Here's the drawing with two shaded views (mm, measured from the low corner). I have some questions. A direction names the side the tool comes from. Give positions to 0.01 mm unless a question says otherwise; leave off trailing zeros. Loops run counter-clockwise (first coordinate to the right, second up) from the corner with the lowest first, then second, coordinate; pieces in that order, holes last. Notation, with made-up numbers: (39.25, 31) - (92.25, 31) arc R21 cw to (92.25, 59) - close; hole circle Ø6 at (68.5, 85.5). An arc over 180 degrees is marked (long way). Use one line per item in the form item = value.
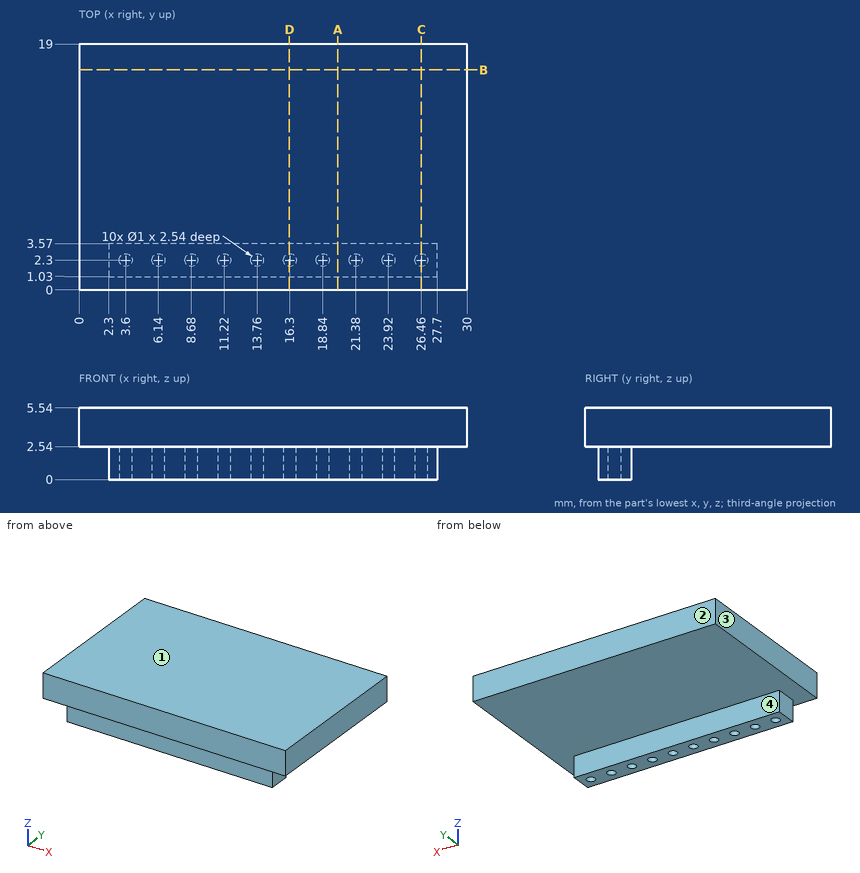
(1) For the marked faces 3 and 4, which set-ups out of +Z, -Z, +X, -X, +Y, -Y let a thin tool reach every point of the face, with its end or its side?
Geometry says:
face_3 = +Z, -Z, -X, +Y, -Y
face_4 = -Z, +X, -X, +Y
(2) If I drill on probe 1 along Y at (x, z) = (13.75, 1.15); probe 2 along Z at (x, y) = (14.75, 7); probe 3 along Y at (x, z) = (23.25, 1.85), over which ranges is the centre line in solid material (lowest first)?
Geometry says:
probe_1 = 1.03 to 1.8, 2.8 to 3.57
probe_2 = 2.54 to 5.54
probe_3 = 1.03 to 3.57
(3) For P1, Ø3, axis at x = 20.5, z = 1, coming from the -Y side; P2, Ø2, axis at y = 1.5, z = 1, coming from the -X side; P3, Ø0.8, axis at x = 10.5, z = 0.5, coming from the +Y side, each with a flat end and sliding along its axis, tell me the tip position at first contact or that it passes through.
Geometry says:
P1 = 1.03
P2 = 2.3
P3 = 3.57
(4) If we section it at C-C (x = 26.46): List the corners of the cut face in (y, z) for me.
Geometry says:
outline = (0, 2.54) - (1.03, 2.54) - (1.03, 0) - (1.8, 0) - (1.8, 2.54) - (2.8, 2.54) - (2.8, 0) - (3.57, 0) - (3.57, 2.54) - (19, 2.54) - (19, 5.54) - (0, 5.54) - close
(5) Thinking about a two-plate mould opening in Z: for the marked faces 1 and 2, which applies, pulls with the +Z half, pulls with the -Z half, needs draft (parallel to the pull), parting line crosses it, or undercut?
Geometry says:
face_1 = pulls with the +Z half
face_2 = needs draft
(6) If we section it at B-B (y = 17): List the corners of the cut face in (x, z) for me, plus the area to 3 significant figures.
Geometry says:
outline = (0, 2.54) - (30, 2.54) - (30, 5.54) - (0, 5.54) - close
area = 90.0 mm²
(7) If we section it at A-A (x = 20): List the corners of the cut face in (y, z) for me.
Geometry says:
outline = (0, 2.54) - (1.03, 2.54) - (1.03, 0) - (3.57, 0) - (3.57, 2.54) - (19, 2.54) - (19, 5.54) - (0, 5.54) - close
